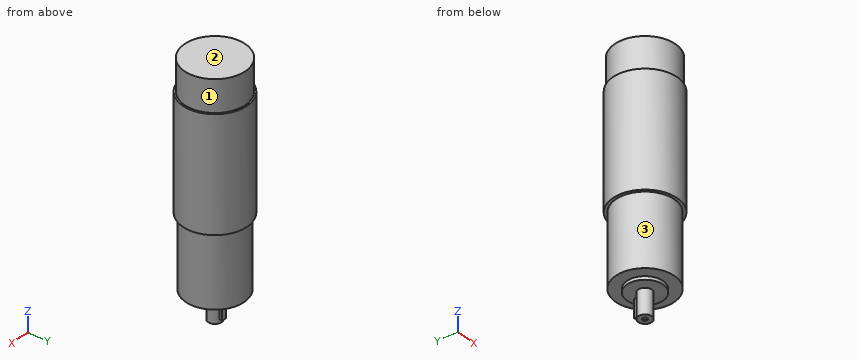
```python
from build123d import *

# Parameters (mm, degrees)
SKETCH2_W           = 16
SKETCH2_H           = 3.081282867
BOSS_EXTRUDE1_DEPTH = 2


with BuildPart() as part:
    # Sketch1 → Revolve1 (revolve)
    with BuildSketch(Plane(origin=(0, 0, 0), x_dir=(0, 0, -1), z_dir=(1, 0, 0)), mode=Mode.PRIVATE) as revolve1_sk:
        Polygon((0, 0), (207.054133767, 0), (208.008, 1.5875), (215.4365, 1.5875), (216.008, 2.159), (216.008, 6), (194.008, 6), (194.008, 16), (191.008, 16), (191.008, 26), (127.837178898, 26), (127.837178898, 28.5), (27.94, 28.5), (27.94, 26.9875), (0, 26.9875), align=None)
    revolve(revolve1_sk.sketch.rotate(Axis((0, 0, 10.8794825), (0, 0, -1)), 90), axis=Axis((0, 0, 10.8794825), (0, 0, -1)))

    # Sketch2 → Boss-Extrude1 (add, symmetric)
    with BuildSketch(Plane(origin=(0, 0, 0), x_dir=(0, 0, -1), z_dir=(1, 0, 0))):
        with Locations((205.008, 6.459358567)):
            Rectangle(SKETCH2_W, SKETCH2_H)
    extrude(amount=BOSS_EXTRUDE1_DEPTH, both=True)


solid = part.part
```
Check sheet for the modelled part. Datum: model origin and axes. Units: mm. Face numbers are marked on the shaded views. A direction names the side the tool comes from. Round coordinates to 2 decimals unless told otherwise and drop trailing zeros. Order: outer loops, then holes, each group sorted by start corner. A loop starts at its lowest first (then second) coordinate and runs counter-clockwise, first axis right, second up. Notation, with made-up numbers: (-36.5, 89) - (16.5, 89) arc R26 cw to (16.5, 112) - close; hole circle Ø10 at (-20.5, -26). An arc over 180 degrees is marked (long way). Write item = value, one per line.
Q1. Section check B-B (y = -12.5). Record the boundary of the cut face in (x, z).
Computed:
outline = (-25.61, -127.84) - (-22.8, -127.84) - (-22.8, -191.01) - (-9.99, -191.01) - (-9.99, -194.01) - (9.99, -194.01) - (9.99, -191.01) - (22.8, -191.01) - (22.8, -127.84) - (25.61, -127.84) - (25.61, -27.94) - (23.92, -27.94) - (23.92, 0) - (-23.92, 0) - (-23.92, -27.94) - (-25.61, -27.94) - close
Q2. Section check C-C (x = -8). Record the boundary of the cut face in (y, z).
Computed:
outline = (-27.35, -127.84) - (-24.74, -127.84) - (-24.74, -191.01) - (-13.86, -191.01) - (-13.86, -194.01) - (13.86, -194.01) - (13.86, -191.01) - (24.74, -191.01) - (24.74, -127.84) - (27.35, -127.84) - (27.35, -27.94) - (25.77, -27.94) - (25.77, 0) - (-25.77, 0) - (-25.77, -27.94) - (-27.35, -27.94) - close
Q3. Section check A-A (z = -73.5). Record the boundary of the cut face in (x, y).
Computed:
outline = circle Ø57 at (0, 0)
Q4. Go/stop test with flat-tipped pins: pin 1 (2 mm diameter, centred on x = -7.5, z = -137, fed in from +Y); pin 2 (6 mm diameter, centred on x = -22.5, y = 14, fed in from -Z); pin 3 (3 mm diameter, centred on y = -2.5, z = -61, fed in from -X). Record where each tip stops, or that it passes through.
Computed:
pin_1 = 25.17
pin_2 = -191.01
pin_3 = -28.48
Q5. Tool access check on the marked faces 1, 2 and 3. Record the directions out of +Z, -Z, +X, -X, +Y, -Y that give a thin tool (end or side, any length) a straight path to the whole face; none if there is none.
Computed:
face_1 = +Z
face_2 = +Z, +X, -X, +Y, -Y
face_3 = -Z
Q6. Thickness scan on line 1 along Y through (x, z) = (0, -210.5); line 2 along Z through (x, y) = (-2.5, 11); line 3 along Z through (x, y) = (-22, -11). Record the ranges inside material, lowest first.
Computed:
line_1 = -6 to -1.59, 1.59 to 8
line_2 = -194.01 to 0
line_3 = -191.01 to 0
Q7. Section check D-D (y = 18). Record the boundary of the cut face in (x, z), and give its area (3 significant figures).
Computed:
outline = (-22.1, -127.84) - (-18.76, -127.84) - (-18.76, -191.01) - (18.76, -191.01) - (18.76, -127.84) - (22.1, -127.84) - (22.1, -27.94) - (20.11, -27.94) - (20.11, 0) - (-20.11, 0) - (-20.11, -27.94) - (-22.1, -27.94) - close
area = 7,910 mm^2
